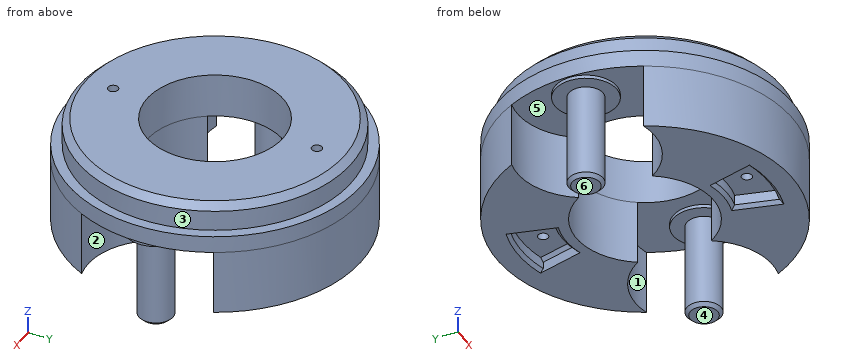
```python
from build123d import *

# Parameters (mm, degrees)
CHAMFER1_SIZE                = 1
SKETCH3_R                    = 4.5
BOSS_EXTRUDE2_DEPTH          = 0.5
SKETCH4_R                    = 2.5
BOSS_EXTRUDE3_DEPTH          = 14
CHAMFER2_SIZE                = 0.5
CIRPATTERN1_COUNT            = 2
CHAMFER2_OF_CIRPATTERN1_SIZE = 0.5
BOSS_EXTRUDE4_DEPTH          = 9.5
SKETCH6_R                    = 0.75
CUT_EXTRUDE2_DEPTH           = 2
SKETCH6_3_R                  = 0.75
CUT_EXTRUDE3_DEPTH           = 35.358405085
CHAMFER3_SIZE                = 0.5
CIRPATTERN2_COUNT            = 2
CHAMFER3_OF_CIRPATTERN2_SIZE = 0.5


with BuildPart() as part:
    # Sketch1 → Revolve1 (revolve)
    with BuildSketch(Plane(origin=(0, 0, 0), x_dir=(0, 0, -1), z_dir=(1, 0, 0)), mode=Mode.PRIVATE) as revolve1_sk:
        Polygon((0, 20), (0, 10), (6.5, 10), (6.5, 13.235638921), (6.5, 20.468347011), (6.5, 21.5), (4, 21.5), (4, 20), align=None)
    revolve(revolve1_sk.sketch.rotate(Axis((0, 0, 0), (0, 0, 1)), 90), axis=Axis((0, 0, 0), (0, 0, 1)))

    # Chamfer1
    chamfer1_edges = [part.edges().sort_by_distance(p)[0] for p in [
        (20, 0, 0),
    ]]
    chamfer(chamfer1_edges, length=CHAMFER1_SIZE)

    # Sketch3 → Boss-Extrude2 (add)
    with BuildSketch(Plane(origin=(0, 0, -6.5), x_dir=(-1, 0, 0), z_dir=(0, 0, -1))):
        with Locations((16.8, 0)):
            Circle(SKETCH3_R)
    boss_extrude2 = extrude(amount=BOSS_EXTRUDE2_DEPTH)

    # Sketch4 → Boss-Extrude3 (add)
    with BuildSketch(Plane(origin=(0, 0, -7), x_dir=(-1, 0, 0), z_dir=(0, 0, -1))):
        with Locations((16.8, 0)):
            Circle(SKETCH4_R)
    boss_extrude3 = extrude(amount=BOSS_EXTRUDE3_DEPTH)

    # Chamfer2
    chamfer2_edges = [part.edges().sort_by_distance(p)[0] for p in [
        (-14.3, 0, -21),
    ]]
    chamfer(chamfer2_edges, length=CHAMFER2_SIZE)

    # CirPattern1: Boss-Extrude2, Boss-Extrude3 ×2 about axis
    cirpattern1_axis = Axis((0, 0, 0), (0, 0, 1))
    add([boss_extrude2.rotate(cirpattern1_axis, i * 360 / CIRPATTERN1_COUNT) for i in range(1, CIRPATTERN1_COUNT)])
    add([boss_extrude3.rotate(cirpattern1_axis, i * 360 / CIRPATTERN1_COUNT) for i in range(1, CIRPATTERN1_COUNT)])

    # Chamfer2 of CirPattern1
    chamfer2_of_cirpattern1_edges = [part.edges().sort_by_distance(p)[0] for p in [
        (14.3, 0, -21),
    ]]
    chamfer(chamfer2_of_cirpattern1_edges, length=CHAMFER2_OF_CIRPATTERN1_SIZE)

    # Sketch5 → Boss-Extrude4 (add)
    with BuildSketch(Plane(origin=(0, 0, -6.5), x_dir=(-1, 0, 0), z_dir=(0, 0, -1))):
        with BuildLine():
            ThreePointArc((-8.4, -5.425863987), (-13.105433977, -9.292479858), (-19.18125, -9.712345156))
            ThreePointArc((-19.18125, -9.712345156), (0, -21.5), (19.18125, -9.712345156))
            ThreePointArc((19.18125, -9.712345156), (13.105433977, -9.292479858), (8.4, -5.425863987))
            ThreePointArc((8.4, -5.425863987), (0, -10), (-8.4, -5.425863987))
        make_face()
    boss_extrude4 = extrude(amount=BOSS_EXTRUDE4_DEPTH)

    # Sketch6 → Cut-Extrude2 (cut)
    # profile 1 of 2: a face of its own
    with BuildSketch(Plane(origin=(0, 0, -16), x_dir=(-1, 0, 0), z_dir=(0, 0, -1))):
        with BuildLine():
            ThreePointArc((3.105828541, -11.591109915), (0, -12), (-3.105828541, -11.591109915))
            Line((-3.105828541, -11.591109915), (-4.658742812, -17.386664873))
            ThreePointArc((-4.658742812, -17.386664873), (0, -18), (4.658742812, -17.386664873))
            Line((4.658742812, -17.386664873), (3.105828541, -11.591109915))
        make_face()
        with Locations((0, -15)):
            Circle(SKETCH6_R, mode=Mode.SUBTRACT)
    # profile 2 of 2: a face of its own
    with BuildSketch(Plane(origin=(0, 0, -16), x_dir=(-1, 0, 0), z_dir=(0, 0, -1))):
        with Locations((0, -15)):
            Circle(SKETCH6_R)
    cut_extrude2 = extrude(amount=-CUT_EXTRUDE2_DEPTH, mode=Mode.SUBTRACT)

    # Sketch6<3> → Cut-Extrude3 (cut, through all)
    with BuildSketch(Plane(origin=(0, 0, -16), x_dir=(-1, 0, 0), z_dir=(0, 0, -1))):
        with Locations((0, -15)):
            Circle(SKETCH6_3_R)
    cut_extrude3 = extrude(amount=-CUT_EXTRUDE3_DEPTH, mode=Mode.SUBTRACT)

    # Chamfer3
    chamfer3_edges = [part.edges().sort_by_distance(p)[0] for p in [
        (0, -12, -16),
        (-3.882285677, -14.488887394, -14),
        (3.882285677, -14.488887394, -16),
        (0, -18, -16),
    ]]
    chamfer(chamfer3_edges, length=CHAMFER3_SIZE)

    # CirPattern2: Boss-Extrude4, Cut-Extrude2, Cut-Extrude3 ×2 about axis
    cirpattern2_axis = Axis((0, 0, 0), (0, 0, 1))
    add([boss_extrude4.rotate(cirpattern2_axis, i * 360 / CIRPATTERN2_COUNT) for i in range(1, CIRPATTERN2_COUNT)])
    add([cut_extrude2.rotate(cirpattern2_axis, i * 360 / CIRPATTERN2_COUNT) for i in range(1, CIRPATTERN2_COUNT)], mode=Mode.SUBTRACT)
    add([cut_extrude3.rotate(cirpattern2_axis, i * 360 / CIRPATTERN2_COUNT) for i in range(1, CIRPATTERN2_COUNT)], mode=Mode.SUBTRACT)

    # Chamfer3 of CirPattern2
    chamfer3_of_cirpattern2_edges = [part.edges().sort_by_distance(p)[0] for p in [
        (0, 12, -16),
        (3.882285677, 14.488887394, -14),
        (-3.882285677, 14.488887394, -16),
        (0, 18, -16),
    ]]
    chamfer(chamfer3_of_cirpattern2_edges, length=CHAMFER3_OF_CIRPATTERN2_SIZE)


solid = part.part
```
Here's how the part is built. I have some questions about the finished solid (model axes, mm). Face numbers are marked on the shaded views. A direction names the side the tool comes from. Round coordinates to 2 decimals unless told otherwise and drop trailing zeros. Order: outer loops, then holes, each group sorted by start corner. A loop starts at its lowest first (then second) coordinate and runs counter-clockwise, first axis right, second up. Notation, with made-up numbers: M 73.25,45 L 127.25,45 A25 cw 127.25,60 Z; hole C 51.5,-15 d1. An arc over 180 degrees is marked long. Answer as CSV lines item,"result".
Item 1: Imagine slicing it at C-C on z = -2.75. List the corners of the cut face in (x, y) for me, and give its area (3 significant figures).
From the geometry:
outline,"C 0,0 d40; hole C 0,0 d20; hole C 0,-15 d1.5; hole C 0,15 d1.5"
area,"939 mm2"
Item 2: For pin 1 (3 mm diameter, centred on y = 5, z = -9.5, fed in from -X); pin 2 (1.5 mm diameter, centred on x = -11, y = -8.5, fed in from +Z); pin 3 (2 mm diameter, centred on y = -11, z = -16, fed in from -X); pin 4 (2 mm diameter, centred on y = 17, z = -13.5, fed in from -X), each with a flat end and sliding along its axis, tell me the tip position at first contact or that it passes through.
From the geometry:
pin 1,"x = -9.2"
pin 2,"z = 0"
pin 3,"x = -19.03"
pin 4,"x = -14.36"
Item 3: Which directions (+Z, -Z, +X, -X, +Y, -Y) give clear straight access to the entire face, cutting with the end or side of a thin tool? Please do the marked faces 5 and 6.
From the geometry:
face 5,"-Z"
face 6,"-Z, +X, -X, +Y, -Y"
Item 4: Imagine slicing it at A-A on z = -10.25. List the corners of the cut face in (x, y) for me.
From the geometry:
outline,"C -16.8,0 d5; M -19.18,-9.71 A21.5 ccw 19.18,-9.71 A10 cw 8.4,-5.43 A10 cw -8.4,-5.43 A10 cw Z; M -19.18,9.71 A10 cw -8.4,5.43 A10 cw 8.4,5.43 A10 cw 19.18,9.71 A21.5 ccw Z; C 16.8,0 d5; hole C 0,-15 d1.5; hole C 0,15 d1.5"
Item 5: Please list where these lines run through material, in increasing order: L1, parallel to Y at x = 0, z = -3.25; L2, parallel to Y at x = 0, z = -5; L3, parallel to Y at x = 15, z = -12.5. Write a range as [from, to].
From the geometry:
L1,"[-20, -15.75], [-14.25, -10], [10, 14.25], [15.75, 20]"
L2,"[-21.5, -15.75], [-14.25, -10], [10, 14.25], [15.75, 21.5]"
L3,"[-15.4, -9.84], [-1.73, 1.73], [9.84, 15.4]"
Item 6: We'd pull the mould along X, two halves only. Please class the marked faces 1, 2, 3 and 4: +X half, -X half, draft (parallel to the pull), parting line (faces both ways), or undercut.
From the geometry:
face 1,"undercut"
face 2,"undercut"
face 3,"parting line"
face 4,"draft"
